Can you work these out from the model? Positions are in its coordinate system, mm. Coordinates: 2 decimals unless noted, no trailing zeros. Order: outer loops, then holes, each group sorted by start corner. A loop starts at its lowest first (then second) coordinate and runs counter-clockwise, first axis right, second up.
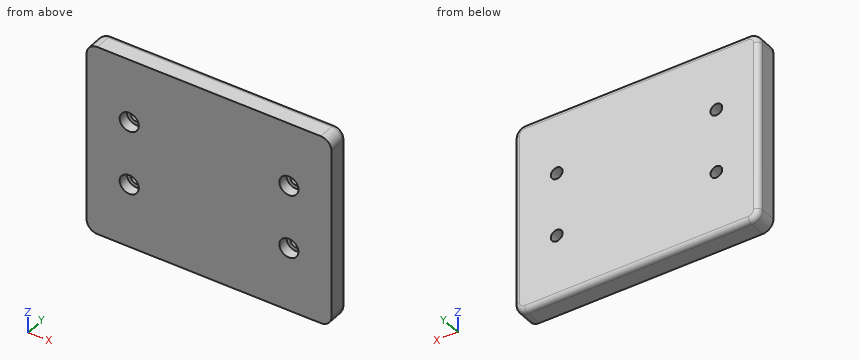
```python
from build123d import *

# Parameters (mm, degrees)
SKETCH1_R            = 11
BOSS_EXTRUDE1_DEPTH  = 40
FILLET1_R            = 10
SKETCH2_R            = 18
CUT_EXTRUDE1_DEPTH   = 20
LPATTERN1_COUNT      = 2
LPATTERN1_PITCH      = 300
LPATTERN1_COUNT_DIR2 = 2
LPATTERN1_PITCH_DIR2 = 120


with BuildPart() as part:
    # Sketch1 → Boss-Extrude1 (new body)
    with BuildSketch(Plane(origin=(0, 0, 0), x_dir=(1, 0, 0), z_dir=(0, 1, 0))):
        with BuildLine():
            Line((-210, -180), (210, -180))
            ThreePointArc((210, -180), (224.142135624, -174.142135624), (230, -160))
            Line((230, -160), (230, 160))
            ThreePointArc((230, 160), (224.142135624, 174.142135624), (210, 180))
            Line((210, 180), (-210, 180))
            ThreePointArc((-210, 180), (-224.142135624, 174.142135624), (-230, 160))
            Line((-230, 160), (-230, -160))
            ThreePointArc((-230, -160), (-224.142135624, -174.142135624), (-210, -180))
        make_face()
        with Locations((-150, 60)):
            Circle(SKETCH1_R, mode=Mode.SUBTRACT)
        with Locations((-150, -60)):
            Circle(SKETCH1_R, mode=Mode.SUBTRACT)
        with Locations((150, -60)):
            Circle(SKETCH1_R, mode=Mode.SUBTRACT)
        with Locations((150, 60)):
            Circle(SKETCH1_R, mode=Mode.SUBTRACT)
    extrude(amount=BOSS_EXTRUDE1_DEPTH)

    # Fillet1
    fillet1_edges = [part.edges().sort_by_distance(p)[0] for p in [
        (224.142135624, 40, 174.142135624),
        (230, 40, 0),
        (224.142135624, 40, -174.142135624),
        (0, 40, -180),
        (-224.142135624, 40, -174.142135624),
        (-230, 40, 0),
        (-224.142135624, 40, 174.142135624),
        (0, 40, 180),
    ]]
    fillet(fillet1_edges, radius=FILLET1_R)

    # Sketch2 → Cut-Extrude1 (cut)
    with BuildSketch(Plane.XZ):
        with Locations((-150, 60)):
            Circle(SKETCH2_R)
    cut_extrude1 = extrude(amount=-CUT_EXTRUDE1_DEPTH, mode=Mode.SUBTRACT)

    # LPattern1: Cut-Extrude1 2 × 2
    with Locations(*[(i * LPATTERN1_PITCH, 0, -j * LPATTERN1_PITCH_DIR2) for i in range(LPATTERN1_COUNT) for j in range(LPATTERN1_COUNT_DIR2) if (i, j) != (0, 0)]):
        add(cut_extrude1, mode=Mode.SUBTRACT)


solid = part.part
```
1. Imagine slicing it at B-B on x = 150. Please give me the cut outline in (y, z).
Completed:
outline: (0, -180) - (30, -180) arc R10 ccw to (40, -170) - (40, -71) - (20, -71) - (20, -78) - (0, -78) - close; (0, -42) - (20, -42) - (20, -49) - (40, -49) - (40, 49) - (20, 49) - (20, 42) - (0, 42) - close; (0, 78) - (20, 78) - (20, 71) - (40, 71) - (40, 170) arc R10 ccw to (30, 180) - (0, 180) - close
2. Imagine slicing it at C-C on y = 10. Please give me the cut outline in (x, z), then the cut area to 3 significant figures.
Completed:
outline: (-230, -160) arc R20 ccw to (-210, -180) - (210, -180) arc R20 ccw to (230, -160) - (230, 160) arc R20 ccw to (210, 180) - (-210, 180) arc R20 ccw to (-230, 160) - close; hole circle Ø36 at (-150, -60); hole circle Ø36 at (-150, 60); hole circle Ø36 at (150, -60); hole circle Ø36 at (150, 60)
area: 161,000 mm2
3. Imagine slicing it at A-A on z = 60. Please give me the cut outline in (x, y), then the cut area to 3 significant figures.
Completed:
outline: (-230, 0) - (-168, 0) - (-168, 20) - (-161, 20) - (-161, 40) - (-220, 40) arc R10 ccw to (-230, 30) - close; (-139, 20) - (-132, 20) - (-132, 0) - (132, 0) - (132, 20) - (139, 20) - (139, 40) - (-139, 40) - close; (161, 20) - (168, 20) - (168, 0) - (230, 0) - (230, 30) arc R10 ccw to (220, 40) - (161, 40) - close
area: 16,000 mm2
4. Please list where these lines run through material, in increasing order: probe 1 along Z at (x, y) = (-150, 10.5); probe 2 along Z at (x, y) = (-150, 30); probe 3 along X at (y, z) = (24, -60).
Completed:
probe 1: z = -180 to -78, -42 to 42, 78 to 180
probe 2: z = -180 to -71, -49 to 49, 71 to 180
probe 3: x = -230 to -161, -139 to 139, 161 to 230
5. I'm going to push flat-ended pins straight in: pin 1 (1 mm diameter, centred on x = 70.5, z = 62.5, fed in from -Y); pin 2 (11 mm diameter, centred on x = -149, z = -51.5, fed in from -Y); pin 3 (20 mm diameter, centred on x = -150, z = -60, fed in from +Y). Where does each tip first touch, or does it pass through?
Completed:
pin 1: stops at y = 0
pin 2: stops at y = 20
pin 3: passes through
